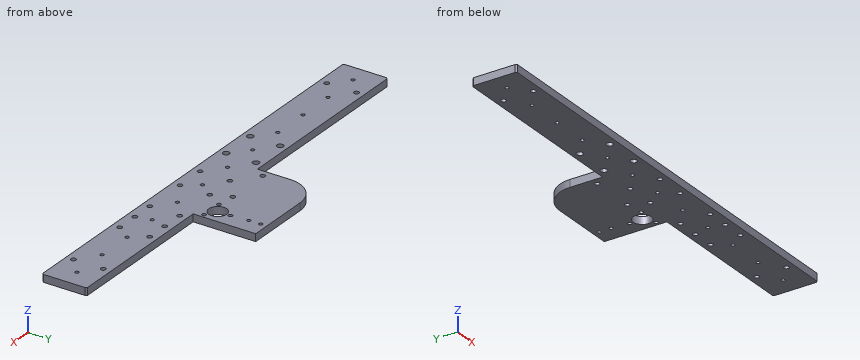
from build123d import *

# Parameters (mm, degrees)
SKETCH_1_W                 = 300
SKETCH_1_H                 = 30
EXTRUDE_1_DEPTH            = 5
CHAMFER_1_SIZE             = 1
HOLE_WIZARD_M3_1_D         = 3.2
M3X0_5_1_D                 = 2.5
M4X0_7_1_D                 = 3.3
M4X0_7_2_D                 = 3.3
PATTERN_LINEAR_1_COUNT     = 6
PATTERN_LINEAR_1_PITCH     = 25
PATTERN_LINEAR_1_COL_COUNT = 7
PATTERN_LINEAR_1_COL_PITCH = 25
EXTRUDE_3_DEPTH            = 5
SKETCH_13_R                = 6
CUT_EXTRUDE_2_DEPTH        = 161.542829177
HOLE_WIZARD_M2_5_1_D       = 2.7
M4X0_7_3_D                 = 3.3
HOLE_WIZARD_M4_1_D         = 4.3
M3X0_5_2_D                 = 2.5
PATTERN_CIRCULAR_1_COUNT   = 3


with BuildPart() as part:
    # 草圖1 → 填料-伸長1 (new body)
    with BuildSketch(Plane.XY):
        Rectangle(SKETCH_1_W, SKETCH_1_H)
    extrude(amount=EXTRUDE_1_DEPTH)

    # 導角1
    chamfer_1_edges = [part.edges().sort_by_distance(p)[0] for p in [
        (150, -15, 2.5),
        (-150, -15, 2.5),
        (-150, 15, 2.5),
        (150, 15, 2.5),
    ]]
    chamfer(chamfer_1_edges, length=CHAMFER_1_SIZE)

    # M3 餘隙孔1 (through all)
    with Locations(Plane.XY.offset(5)):
        with Locations((20, -10), (20, 10), (0, -10), (0, 10)):
            Hole(HOLE_WIZARD_M3_1_D / 2)

    # M3x0.5 螺紋孔1 (through all)
    with Locations(Plane.XY.offset(5)):
        with Locations((-12.5, 0)):
            m3x0_5_1 = Hole(M3X0_5_1_D / 2)

    # M4x0.7 螺紋孔1 (through all)
    with Locations(Plane.XY.offset(5)):
        with Locations((80, 10), (50, -10), (50, 10), (80, -10), (65, 10), (65, -10)):
            Hole(M4X0_7_1_D / 2)

    # M4x0.7 螺紋孔2 (through all)
    with Locations(Plane.XY.offset(5)):
        with Locations((-126, 10), (-126, -10)):
            m4x0_7_2 = Hole(M4X0_7_2_D / 2)

    # 直線複製排列1: M3x0.5 螺紋孔1 ×6
    with Locations(*[(-i * PATTERN_LINEAR_1_PITCH, 0, 0) for i in range(1, PATTERN_LINEAR_1_COUNT)]):
        add(m3x0_5_1, mode=Mode.SUBTRACT)

    # 直線複製排列1 col: M3x0.5 螺紋孔1 ×7
    with Locations(*[(i * PATTERN_LINEAR_1_COL_PITCH, 0, 0) for i in range(1, PATTERN_LINEAR_1_COL_COUNT)]):
        add(m3x0_5_1, mode=Mode.SUBTRACT)

    # 鏡射1: M4x0.7 螺紋孔2 across plane
    add(m4x0_7_2.mirror(Plane(origin=(0, 0, 0), x_dir=(0, 0, 1), z_dir=(1, 0, 0))), mode=Mode.SUBTRACT)

    # 草圖16 → 填料-伸長3 (add, through all)
    with BuildSketch(Plane.XY):
        with BuildLine():
            Line((-20, 15), (44, 15))
            Line((44, 15), (44, 57))
            Line((44, 57), (0, 57))
            ThreePointArc((0, 57), (-14.142135624, 51.142135624), (-20, 37))
            Line((-20, 37), (-20, 15))
        make_face()
    extrude(amount=EXTRUDE_3_DEPTH)

    # 草圖13 → 除料-伸長2 (cut, through all)
    with BuildSketch(Plane.XY):
        with Locations(Location((34, 24.8, 0), (0, 0, 180))):
            Circle(SKETCH_13_R)
    extrude(amount=CUT_EXTRUDE_2_DEPTH, mode=Mode.SUBTRACT)

    # M2.5 餘隙孔1 (through all)
    with Locations(Plane.XY.offset(5)):
        with Locations((34, 33.3)):
            hole_wizard_m2_5_1 = Hole(HOLE_WIZARD_M2_5_1_D / 2)

    # M4x0.7 螺紋孔3 (through all)
    with Locations(Plane.XY.offset(5)):
        with Locations((15, 22), (-15, 22)):
            Hole(M4X0_7_3_D / 2)

    # M4 餘隙孔1 (through all)
    with Locations(Plane.XY.offset(5)):
        with Locations((-26, -10), (-26, 10), (-50, -10), (-50, 10)):
            Hole(HOLE_WIZARD_M4_1_D / 2)

    # M3x0.5 螺紋孔2 (through all)
    with Locations(Plane.XY.offset(5)):
        with Locations((33, 53), (33, 45)):
            Hole(M3X0_5_2_D / 2)

    # 環狀複製排列1: M2.5 餘隙孔1 ×3 about axis
    pattern_circular_1_axis = Axis((34, 24.8, 0), (0, 0, 1))
    for i in range(1, PATTERN_CIRCULAR_1_COUNT):
        add(hole_wizard_m2_5_1.rotate(pattern_circular_1_axis, i * 360 / PATTERN_CIRCULAR_1_COUNT), mode=Mode.SUBTRACT)


solid = part.part
The listing builds one solid part. Answer for the finished solid, in the listing's coordinates (mm). Give positions to 0.01 mm unless a question says otherwise; leave off trailing zeros. Loops run counter-clockwise (first coordinate to the right, second up) from the corner with the lowest first, then second, coordinate; pieces in that order, holes last.
Item 1: Find the intervals of material crossed by line 1 along Y through (x, z) = (20, 3.2); line 2 along Y through (x, z) = (-50, 1.75); line 3 along Y through (x, z) = (-110.5, 0.35), in increasing order.
Derived:
line 1: y = -15 to -11.6, -8.4 to 8.4, 11.6 to 57
line 2: y = -15 to -12.15, -7.85 to 7.85, 12.15 to 15
line 3: y = -15 to 15
Item 2: A cutting plane is placed at A-A (x = -91.5). Give the vertices of the cut face in (y, z), then the cut area to 3 significant figures.
Derived:
outline: (-15, 0) - (15, 0) - (15, 5) - (-15, 5) - close
area: 150 mm2
Item 3: Each of these flat-tipped pins is pushed along its axis until it touches: pin 1 Ø2.5 at (x, y) = (20, -10) entering from +Z; pin 2 Ø1.5 at (y, z) = (40.5, 2) entering from +X; pin 3 Ø3 at (x, z) = (-31, 0.5) entering from +Y. Where does it stop, or does it pass through?
Derived:
pin 1: passes through
pin 2: stops at x = 44
pin 3: stops at y = 15
Item 4: A cutting plane is placed at B-B (z = 1.25). Give the number of separate pieces and of enclosed holes in the cut face, then the cut area to 3 significant figures.
Derived:
separate pieces: 1
enclosed holes: 38
area: 11,200 mm2
